Autodesk Inventor part; units mm, degrees
ref_plane "YZ Plane" through (0, 0, 0) normal (1, 0, 0) x (0, 1, 0)
ref_plane "XZ Plane" through (0, 0, 0) normal (0, 1, 0) x (-1, 0, 0)
ref_plane "XY Plane" through (0, 0, 0) normal (0, 0, 1) x (1, 0, 0)
sketch "Sketch1" plane through (0, 0, 0) normal (0, 1, 0) x (-1, 0, 0)
  line L0 (-1.8331, -3.175) -> (-3.6662, 0)
  line L1 (-3.6662, 0) -> (-1.8331, 3.175)
  line L2 (-1.8331, 3.175) -> (1.8331, 3.175)
  line L3 (1.8331, 3.175) -> (3.6662, 0)
  line L4 (3.6662, 0) -> (1.8331, -3.175)
  line L5 (1.8331, -3.175) -> (-1.8331, -3.175)
  point P0 (0, 0)
  point P1 (0, 0)
  dimension "d0" = 6.35
extrude "Body" add sketch "Sketch1" along normal blind 6.35
sketch "Sketch2" plane through (0, 6.35, 0) normal (0, 1, 0) x (1, 0, 0)
  circle A0 centre (0, 0) radius 2.0955
  dimension "d3" = 4.191
extrude "Hole 2" [suppressed]
sketch "Sketch3" plane through (0, 0, 0) normal (0, -1, 0) x (1, 0, 0)
  circle A0 centre (0, 0) radius 2.0955
  dimension "d6" = 4.191
extrude "Hole 1" cut sketch "Sketch3" against normal blind 12.7
chamfer "Hole 2 Chamfer 1" [suppressed]
chamfer "Hole 1 Chamfer 1" distance 0.127 distance2 0.1244 1 edges at (-2.0955, 0, 0) measured on face at (-0.0842, 0, 2.8101)
sketch "Sketch4" plane through (0, 0, 0) normal (0, 0, 1) x (1, 0, 0)
  line L0 (1.8331, 6.35) -> (-1.8331, 6.35)
  line L1 (0, 6.35) -> (-3.0353, 6.35)
  line L2 (-3.6662, 6.35) -> (-1.8331, 6.35)
  line L3 (-3.6662, 0) -> (-3.6662, 6.35)
  arc A0 (-3.0353, 6.35) -> (-3.6662, 5.715) centre (-2.2234, 4.9124) ccw
  line L4 (-3.6662, 5.715) -> (-6.3588, 8.3147)
  line L5 (-6.3588, 8.3147) -> (0, 6.35)
  line L6 (0, 6.35) -> (0, 2.864)
  point P0 (0, 0)
  dimension "d15" = 3.0353
  dimension "d16" = 1.651
  dimension "d17" = 0.635
revolve "Hole 2 Chamfer 2" [suppressed]
sketch "Sketch5" plane through (0, 0, 0) normal (0, 0, 1) x (1, 0, 0)
  line L0 (0, 0) -> (-3.0353, 0)
  line L1 (1.8331, 0) -> (-1.8331, 0)
  line L2 (-3.6662, 0) -> (-3.6662, 6.35)
  arc A0 (-3.6662, 0.635) -> (-3.0353, 0) centre (-2.2234, 1.4376) ccw
  line L3 (0, 0) -> (0, -2.1986)
  line L4 (-3.6662, 0.635) -> (-4.1154, -0.8715)
  line L5 (-4.1154, -0.8715) -> (0, 0)
  point P0 (-3.6662, 151.765)
  dimension "d19" = 3.0353
  dimension "d20" = 1.651
  dimension "d21" = 0.635
revolve "Hole 1 Chamfer 2" cut sketch "Sketch5" angle 360 about axis through (0, 0, 0) along (0, -1, 0)
chamfer "Hole 2 Chamfer 1 For Short" distance 0.127 distance2 0.1244 1 edges at (-2.0955, 6.35, 0) measured on face at (-0.0842, 6.35, 2.8101)
sketch "Sketch7" plane through (0, 0, 0) normal (0, 0, 1) x (1, 0, 0)
  line L0 (0.0002, 6.3504) -> (3.0355, 6.35)
  line L1 (3.6662, 6.35) -> (1.8331, 6.35)
  line L2 (3.6662, 0.635) -> (3.6662, 6.35)
  arc A0 (3.6662, 5.715) -> (3.0355, 6.35) centre (2.2233, 4.9126) ccw
  line L3 (3.6662, 5.715) -> (4.2665, 7.2532)
  line L4 (4.2665, 7.2532) -> (0.0002, 6.3504)
  line L5 (0.0002, 8.1561) -> (0.0002, 6.3504)
  line L6 (1.8331, 6.35) -> (-1.8331, 6.35)
  point P0 (0, 0)
  dimension "d33" = 3.0353
  dimension "d34" = 1.651
  dimension "d35" = 0.635
revolve "Hole 2 Chamfer 2 For Short" cut sketch "Sketch7" angle 360 about axis through (0.0002, 8.1561, 0) along (0, -1, 0)
properties part number "Standoff .25" material "VEX Aluminum Alloy 5052-H32"
The listing builds one solid part. Answer for the finished solid, in the listing's coordinates (mm). Coordinates: 2 decimals unless noted, no trailing zeros. Write each loop counter-clockwise with the first axis right and the second up, starting at its lowest first coordinate (ties: lowest second). Pieces come first, ordered by that corner, then holes.
Q1. Section A-A, the plane y = 3.25 is taken. Write down the section's boundary in (x, z) (1 decimal).
Returned:
outline: (-3.7, 0) - (-1.8, -3.2) - (1.8, -3.2) - (3.7, 0) - (1.8, 3.2) - (-1.8, 3.2) - close; hole circle Ø4.2 at (0, 0)
Q2. The mould has two halves that part along Z. Classify faces 1 (the flat face through (2, 0, 2)), 2 (the flat face through (2.76, 3.13, 1.57)), 3 (the cylindrical face through (2, 3.13, 0.63)): released by +Z, released by -Z, zero draft, split by the parting line, or undercut.
Returned:
face 1: zero draft
face 2: released by +Z
face 3: undercut
Q3. Find the intervals of material crossed by line 1 along Z through (x, y) = (0, 3.75) (1 decimal); line 2 along X through (y, z) = (5, 0.5); line 3 along X through (y, z) = (1.5, 2.5), in increasing order.
Returned:
line 1: z = -3.2 to -2.1, 2.1 to 3.2
line 2: x = -3.38 to -2.03, 2.03 to 3.38
line 3: x = -2.22 to 2.22
Q4. Given P1, Ø1.5, axis at y = 1.5, z = 2, coming from the +X side, flat-ended and moving along its own axis, determine where the tip first touches the part or whether it passes through.
Returned:
P1: stops at x = 2.94
